```python
from build123d import *

# Parameters (mm, degrees)
SKETCH1_W           = 8.5
SKETCH1_H           = 12
SKETCH1_R           = 1.6
BOSS_EXTRUDE1_DEPTH = 2.8
CUT_EXTRUDE1_DEPTH  = 2.5
SKETCH3_W           = 0.75
SKETCH3_H           = 0.55
BOSS_EXTRUDE2_DEPTH = 13
BOSS_EXTRUDE3_DEPTH = 0.55
SKETCH5_W           = 6
SKETCH5_H           = 8
SKETCH5_R           = 1.6
BOSS_EXTRUDE4_DEPTH = 0.001


with BuildPart() as part:
    # Sketch1 → Boss-Extrude1 (new body)
    with BuildSketch(Plane.XY):
        with Locations((4.25, -6)):
            Rectangle(SKETCH1_W, SKETCH1_H)
        with Locations((4.25, -3.8)):
            Circle(SKETCH1_R, mode=Mode.SUBTRACT)
    extrude(amount=BOSS_EXTRUDE1_DEPTH)

    # Sketch2 → Cut-Extrude1 (cut)
    with BuildSketch(Plane.XY.offset(2.8)):
        with BuildLine():
            Line((2.321539031, -5.259807621), (3.038934241, -4.845619303))
            ThreePointArc((3.038934241, -4.845619303), (2.864359354, -4.6), (2.738934241, -4.326004061))
            Line((2.738934241, -4.326004061), (2.021539031, -4.740192379))
            Line((2.021539031, -4.740192379), (2.321539031, -5.259807621))
        make_face()
        with BuildLine():
            Line((6.178460969, -5.259807621), (6.478460969, -4.740192379))
            Line((6.478460969, -4.740192379), (5.761065759, -4.326004061))
            ThreePointArc((5.761065759, -4.326004061), (5.635640646, -4.6), (5.461065759, -4.845619303))
            Line((5.461065759, -4.845619303), (6.178460969, -5.259807621))
        make_face()
        with BuildLine():
            ThreePointArc((3.95, -2.228376635), (4.25, -2.2), (4.55, -2.228376635))
            Line((4.55, -2.228376635), (4.55, -1.4))
            Line((4.55, -1.4), (3.95, -1.4))
            Line((3.95, -1.4), (3.95, -2.228376635))
        make_face()
    extrude(amount=-CUT_EXTRUDE1_DEPTH, mode=Mode.SUBTRACT)

    # Sketch3 → Boss-Extrude2 (add)
    with BuildSketch(Plane.XZ.offset(12)):
        with Locations((2.065, 1.519799242)):
            Rectangle(SKETCH3_W, SKETCH3_H)
        with Locations((4.252122452, 1.519799242)):
            Rectangle(SKETCH3_W, SKETCH3_H)
        with Locations((6.439244903, 1.519799242)):
            Rectangle(SKETCH3_W, SKETCH3_H)
    extrude(amount=BOSS_EXTRUDE2_DEPTH)

    # Sketch4 → Boss-Extrude3 (add)
    with BuildSketch(Plane.XY.offset(1.794799242)):
        Polygon((3.652122452, -14), (4.152122452, -14.5), (4.352122452, -14.5), (4.852122452, -14), (4.852122452, -12), (3.652122452, -12), align=None)
    extrude(amount=-BOSS_EXTRUDE3_DEPTH)

    # Sketch5 → Boss-Extrude4 (add)
    with BuildSketch(Plane(origin=(0, 0, 0), x_dir=(-1, 0, 0), z_dir=(0, 0, -1))):
        with Locations((-4.25, -5)):
            Rectangle(SKETCH5_W, SKETCH5_H)
        with Locations((-4.25, -3.8)):
            Circle(SKETCH5_R, mode=Mode.SUBTRACT)
    extrude(amount=BOSS_EXTRUDE4_DEPTH)


solid = part.part
```
Build history of the part. All positions in model axes, mm. A direction names the side the tool comes from. Round coordinates to 2 decimals unless told otherwise and drop trailing zeros. Order: outer loops, then holes, each group sorted by start corner. A loop starts at its lowest first (then second) coordinate and runs counter-clockwise, first axis right, second up. Notation, with made-up numbers: (-32.5, 79) - (12.5, 79) arc R25 ccw to (12.5, 103) - close; hole circle Ø1 at (79, 47.5). An arc over 180 degrees is marked (long way). Use a Markdown table: item, result.
1) Flat gauge pins, fed straight in: pin 1 Ø1 at (x, y) = (2, -16.5) entering from +Z; pin 2 Ø1.5 at (x, z) = (1, 2.5) entering from -Y. Where does each tip first touch, or does it go through?
Recorded:
| item | result |
|---|---|
| pin 1 | stops at z = 1.79 |
| pin 2 | stops at y = -12 |
2) Wall check: L1, parallel to X at y = -18, z = 1.45; L2, parallel to Y at x = 4.25, z = 0.85; L3, parallel to Y at x = 4.25, z = 1.55. Give the ranges that are in metal, low to high.
Recorded:
| item | result |
|---|---|
| L1 | x = 1.69 to 2.44, 3.88 to 4.63, 6.06 to 6.81 |
| L2 | y = -12 to -5.4, -1.4 to 0 |
| L3 | y = -25 to -5.4, -1.4 to 0 |
3) Pull direction X, two halves, no side cores. Call faces 5 (the face through (0, -6, 1)), 6 (the face through (4, -10, 0)), 7 (the face through (4.55, -2, 2)): pulls with the +X half, pulls with the -X half, needs draft (parallel to the pull), parting line crosses it, or undercut.
Recorded:
| item | result |
|---|---|
| face 5 | pulls with the -X half |
| face 6 | needs draft |
| face 7 | undercut |
4) Saw through at A-A on y = -13.5. Write the cut outline in (x, z), and give its area (4 significant figures).
Recorded:
| item | result |
|---|---|
| outline | (1.69, 1.24) - (2.44, 1.24) - (2.44, 1.79) - (1.69, 1.79) - close; (3.65, 1.24) - (4.85, 1.24) - (4.85, 1.79) - (3.65, 1.79) - close; (6.06, 1.24) - (6.81, 1.24) - (6.81, 1.79) - (6.06, 1.79) - close |
| area | 1.485 mm² |
5) Tool access for faces 1 (the face through (4.2, -18.4, 1.795)), 2 (the face through (2.5, -4.8, 0.3)), 3 (the face through (4, -6, -0.001)), 4 (the face through (4.2, -18.4, 1.245)): list every direction of +Z, -Z, +X, -X, +Y, -Y with a clear straight run to the whole face (end or side of a thin tool).
Recorded:
| item | result |
|---|---|
| face 1 | +Z, +X, -X, -Y |
| face 2 | +Z |
| face 3 | -Z, +X, -X, +Y, -Y |
| face 4 | -Z, +X, -X, -Y |
6) Saw through at D-D on x = 7.5. Write the cut outline in (y, z), and give its area (3 significant figures).
Recorded:
| item | result |
|---|---|
| outline | (-12, 0) - (0, 0) - (0, 2.8) - (-12, 2.8) - close |
| area | 33.6 mm² |
